Can you work these out from the model? Positions are in its coordinate system, mm. Face numbers are marked on the shaded views. A direction names the side the tool comes from. Round coordinates to 2 decimals unless told otherwise and drop trailing zeros. Loops run counter-clockwise (first coordinate to the right, second up) from the corner with the lowest first, then second, coordinate; pieces in that order, holes last.
from build123d import *

# Parameters (mm, degrees)
F0_W     = 42
F0_H     = 42
F0_R     = 11
F0_R_2   = 3.5
F1_DEPTH = 8
F2_DEPTH = 2
F3_D     = 3
F4_W     = 27.35
F4_H     = 2
F5_DEPTH = 42
F6_W     = 27.35
F6_H     = 2
F7_DEPTH = 42
F8_SIZE  = 4
F9_SIZE  = 0.5


with BuildPart() as f1:
    # F0 (on Top) → F1 (new body)
    with BuildSketch(Plane.XY):
        Rectangle(F0_W, F0_H)
        Circle(F0_R, mode=Mode.SUBTRACT)
        Circle(F0_R)
        Circle(F0_R_2, mode=Mode.SUBTRACT)
        Circle(F0_R_2)
    extrude(amount=-F1_DEPTH)

    # F0 (on Top) → F2 (join)
    with BuildSketch(Plane.XY):
        Circle(F0_R)
        Circle(F0_R_2, mode=Mode.SUBTRACT)
    extrude(amount=F2_DEPTH)

    # F3 (through all)
    with Locations(Plane.XY):
        with Locations((15.5, 15.5), (15.5, -15.5), (-15.5, -15.5), (-15.5, 15.5)):
            Hole(F3_D / 2)

    # F4 (on face) → F5 (cut, through all)
    with BuildSketch(Plane.XZ.offset(21)):
        with Locations((0, -7)):
            Rectangle(F4_W, F4_H)
    extrude(amount=-F5_DEPTH, mode=Mode.SUBTRACT)

    # F6 (on face) → F7 (cut, through all)
    with BuildSketch(Plane(origin=(-21, 0, 0), x_dir=(0, -1, 0), z_dir=(-1, 0, 0))):
        with Locations((0, -7)):
            Rectangle(F6_W, F6_H)
    extrude(amount=-F7_DEPTH, mode=Mode.SUBTRACT)

    # F8
    f8_edges = [f1.edges().sort_by_distance(p)[0] for p in [
        (-21, -21, -4),
        (-21, 21, -4),
        (21, -21, -4),
        (21, 21, -4),
    ]]
    chamfer(f8_edges, length=F8_SIZE)

    # F9
    f9_edges = [f1.edges().sort_by_distance(p)[0] for p in [
        (-11, 0, 2),
        (-21, 0, 0),
        (-19, -19, 0),
        (0, -21, 0),
        (19, -19, 0),
        (21, 0, 0),
        (19, 19, 0),
        (0, 21, 0),
        (-19, 19, 0),
    ]]
    chamfer(f9_edges, length=F9_SIZE)


solid = f1.part
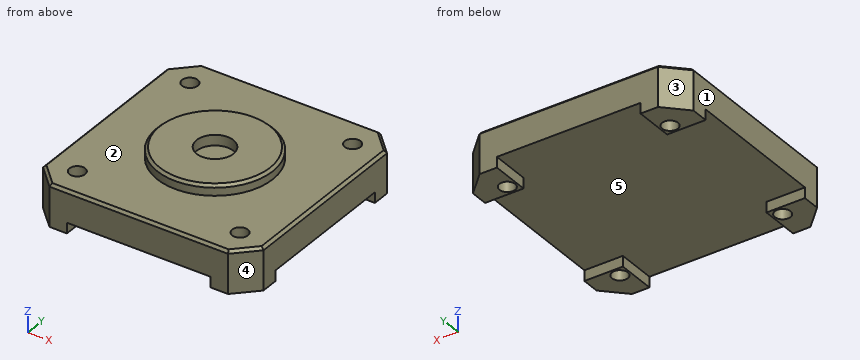
(1) For the marked faces 1 and 2, which set-ups out of +Z, -Z, +X, -X, +Y, -Y let a thin tool reach every point of the face, with its end or its side?
Worked answers:
face 1: +Z, -Z, -X, +Y, -Y
face 2: +Z
(2) If we section it at A-A, the plane x = 15.5: List the corners of the cut face in (y, z) for me (3 decimals), then the cut area to 3 significant figures.
Worked answers:
outline: (-21, -8) - (-17, -8) - (-17, 0) - (-20.5, 0) - (-21, -0.5) - close; (-14, -8) - (-13.675, -8) - (-13.675, -6) - (13.675, -6) - (13.675, -8) - (14, -8) - (14, 0) - (-14, 0) - close; (17, -8) - (21, -8) - (21, -0.5) - (20.5, 0) - (17, 0) - close
area: 233 mm2
(3) If we section it at D-D, the plane x = 0: List the corners of the cut face in (y, z) for me, then the cut area to 4 significant figures.
Worked answers:
outline: (-21, -6) - (21, -6) - (21, -0.5) - (20.5, 0) - (11, 0) - (11, 1.5) - (10.5, 2) - (3.5, 2) - (3.5, 0) - (-3.5, 0) - (-3.5, 2) - (-10.5, 2) - (-11, 1.5) - (-11, 0) - (-20.5, 0) - (-21, -0.5) - close
area: 281.5 mm2
(4) If we section it at C-C, the plane z = -1.75: List the corners of the cut face in (x, y) for me.
Worked answers:
outline: (-21, -17) - (-17, -21) - (17, -21) - (21, -17) - (21, 17) - (17, 21) - (-17, 21) - (-21, 17) - close; hole circle Ø3 at (-15.5, -15.5); hole circle Ø3 at (-15.5, 15.5); hole circle Ø3 at (15.5, -15.5); hole circle Ø3 at (15.5, 15.5)
(5) If we mould it in two halves opening along Y, with no side actions, what happens to the marked faces 3, 4 and 5? For each: released by +Y, released by -Y, zero draft, split by the parting line, or undercut.
Worked answers:
face 3: released by +Y
face 4: released by -Y
face 5: undercut
(6) If I drill on line 1 (Y direction, x = 15.5, z = -3.25); line 2 (X direction, y = -15, z = -6.25) (3 decimals); line 3 (Y direction, x = 0, z = 0.8), over which ranges is the centre line in solid material (lowest first)?
Worked answers:
line 1: y = -21 to -17, -14 to 14, 17 to 21
line 2: x = -21 to -16.914, -14.086 to -13.675, 13.675 to 14.086, 16.914 to 21
line 3: y = -11 to -3.5, 3.5 to 11
(7) Will these pins go through, and if not, where does the flat tip stop? P1, Ø3.5, axis at x = 15.5, y = 15.5, coming from the +Z side; P2, Ø1.6, axis at x = 18, z = -7.5, coming from the -Y side; P3, Ø0.6, axis at y = -19, z = -7, coming from the +X side.
Worked answers:
P1: stops at z = 0
P2: stops at y = -20.8
P3: stops at x = 19.3
